Solid Edge part; units mm, degrees
sketch "Sketch1" plane through (0, 0, 0) normal (0, -1, 0) x (1, 0, 0)
  line L0 (0, 0) -> (115, 0)
  line L1 (115, 0) -> (115, 50)
  line L2 (115, 50) -> (0, 50)
  line L3 (0, 50) -> (0, 0)
  dimension "D1" = 115
extrude "Protrusion1" add sketch "Sketch1" against normal blind 50
fillet "Verrundung_2" radius 20 4 edges at (57.5, 50, 50) (57.5, 50, 0) (57.5, 0, 50) (57.5, 0, 0)
sketch "Sketch2" plane through (0, 25, 25) normal (-1, 0, 0) x (0, 0, -1)
  line L0 (-7.5, -7.5) -> (7.5, -7.5)
  line L1 (7.5, -7.5) -> (7.5, 7.5)
  line L2 (7.5, 7.5) -> (-7.5, 7.5)
  line L3 (-7.5, 7.5) -> (-7.5, -7.5)
  dimension "D1" = 7.5
extrude "Extrusionsausschnitt_5" cut sketch "Sketch2" against normal blind 15
chamfer "Fase_3" distance 2 angle 45 4 edges at (0, 25, 32.5) (0, 17.5, 25) (0, 25, 17.5) (0, 32.5, 25)
sketch "Sketch3" plane through (115, 25, 25) normal (1, 0, 0) x (0, 1, 0)
  line L0 (-7.5, -7.5) -> (7.5, -7.5)
  line L1 (7.5, -7.5) -> (7.5, 7.5)
  line L2 (7.5, 7.5) -> (-7.5, 7.5)
  line L3 (-7.5, 7.5) -> (-7.5, -7.5)
  dimension "D1" = 7.5
extrude "Extrusionsausprägung_2" add sketch "Sketch3" along normal blind 25
sketch "Sketch4" plane through (57.5, 25, 0) normal (0, 0, -1) x (-1, 0, 0)
  line L0 (-47.5, -17.5) -> (32.5, -17.5)
  line L1 (32.5, -17.5) -> (32.5, 17.5)
  line L2 (32.5, 17.5) -> (-47.5, 17.5)
  line L3 (-47.5, 17.5) -> (-47.5, -17.5)
  dimension "D1" = 32.5
  dimension "D2" = 32.5
extrude "Extrusionsausschnitt_6" cut sketch "Sketch4" against normal blind 20
sketch "Sketch5" plane through (65, 25, 20) normal (0, 0, -1) x (-1, 0, 0)
  line L0 (-40, 17.5) -> (40, 17.5)
  line L1 (40, 17.5) -> (40, -17.5)
  line L2 (40, -17.5) -> (-40, -17.5)
  line L3 (-40, -17.5) -> (-40, 17.5)
  line L4 (-34.5, 7) -> (-25.5, 7)
  line L5 (-25.5, 7) -> (-25.5, 16)
  line L6 (-25.5, 16) -> (-34.5, 16)
  line L7 (-34.5, 16) -> (-34.5, 7)
  line L8 (-34.5, -16) -> (-25.5, -16)
  line L9 (-25.5, -16) -> (-25.5, -7)
  line L10 (-25.5, -7) -> (-34.5, -7)
  line L11 (-34.5, -7) -> (-34.5, -16)
  line L12 (23.5, 7) -> (32.5, 7)
  line L13 (32.5, 7) -> (32.5, 16)
  line L14 (32.5, 16) -> (23.5, 16)
  line L15 (23.5, 16) -> (23.5, 7)
  line L16 (23.5, -16) -> (32.5, -16)
  line L17 (32.5, -16) -> (32.5, -7)
  line L18 (32.5, -7) -> (23.5, -7)
  line L19 (23.5, -7) -> (23.5, -16)
extrude "Extrusionsausschnitt_8" cut sketch "Sketch5" against normal blind 5
sketch "Sketch6" plane through (65, 42.5, 14.6938) normal (0, -1, 0) x (-1, 0, 0)
  line L0 (-40, -10.3062) -> (40, -10.3062)
  line L1 (40, -10.3062) -> (40, 10.3062)
  line L2 (40, 10.3062) -> (-40, 10.3062)
  line L3 (-40, 10.3062) -> (-40, -10.3062)
extrude "Extrusionsausschnitt_9" cut sketch "Sketch6" against normal blind 12
sketch "Sketch7" plane through (57.5, 50, 25) normal (0, 1, 0) x (-1, 0, 0)
  line L0 (32.5, 0) -> (45, -25)
  line L1 (45, -25) -> (32.5, -25)
  line L2 (32.5, -25) -> (32.5, 0)
extrude "Cutout1" cut sketch "Sketch7" against normal up to vertex (42.5 mm away)
fillet "Verrundung_3" radius 7.5 2 edges at (140, 25, 17.5) (140, 25, 32.5)
sketch "Sketch8" plane through (127.5, 32.5, 25) normal (0, 1, 0) x (-1, 0, 0)
  circle A0 centre (-5, 0) radius 2.05
extrude "Cutout2" cut sketch "Sketch8" against normal through all
chamfer "Fase_4" distance 1 angle 45 2 edges at (134.55, 32.5, 25) (132.5, 17.5, 22.95)
sketch "Sketch9" plane through (123.75, 25, 17.5) normal (0, 0, -1) x (-1, 0, 0)
  line L0 (8.75, -7.5) -> (8.75, 0)
  line L1 (8.75, 0) -> (-16.25, 0)
  line L2 (-16.25, 0) -> (-16.25, -7.5)
  line L3 (-16.25, -7.5) -> (8.75, -7.5)
extrude "Cutout3" cut sketch "Sketch9" against normal through all
sketch "Sketch10" plane through (95, 36.5, 20) normal (0, 0, -1) x (-1, 0, 0)
  line L0 (-4.5, 4.5) -> (62.5, 4.5)
  line L1 (62.5, 4.5) -> (62.5, -27.5)
  line L2 (62.5, -27.5) -> (-4.5, -27.5)
  line L3 (-4.5, -27.5) -> (-4.5, 4.5)
extrude "Cutout4" cut sketch "Sketch10" against normal up to vertex (5 mm away)
sketch "Sketch11" plane through (65, 28.75, 25) normal (0, 0, -1) x (-1, 0, 0)
  circle A0 centre (30, 13.25) radius 1.2
  circle A1 centre (-28, 13.25) radius 1.2
  circle A2 centre (-28, -9.75) radius 1.2
  circle A3 centre (30, -9.75) radius 1.2
  dimension "D1" = 30
extrude "Extrusionsausschnitt_14" cut sketch "Sketch11" against normal blind 10
sketch "Sketch12" plane through (65, 28.75, 25) normal (0, 0, -1) x (-1, 0, 0)
  line L0 (-31.5, 9.75) -> (-24.5, 9.75)
  line L1 (-24.5, 9.75) -> (-24.5, 16.75)
  line L2 (-24.5, 16.75) -> (-31.5, 16.75)
  line L3 (-31.5, 16.75) -> (-31.5, 9.75)
  line L4 (-31.5, -13.25) -> (-24.5, -13.25)
  line L5 (-24.5, -13.25) -> (-24.5, -6.25)
  line L6 (-24.5, -6.25) -> (-31.5, -6.25)
  line L7 (-31.5, -6.25) -> (-31.5, -13.25)
  line L8 (26.5, -13.25) -> (33.5, -13.25)
  line L9 (33.5, -13.25) -> (33.5, -6.25)
  line L10 (33.5, -6.25) -> (26.5, -6.25)
  line L11 (26.5, -6.25) -> (26.5, -13.25)
  line L12 (26.5, 9.75) -> (33.5, 9.75)
  line L13 (33.5, 9.75) -> (33.5, 16.75)
  line L14 (33.5, 16.75) -> (26.5, 16.75)
  line L15 (26.5, 16.75) -> (26.5, 9.75)
  circle A0 centre (-28, 13.25) radius 1.2
  circle A1 centre (-28, -9.75) radius 1.2
  circle A2 centre (30, -9.75) radius 1.2
  circle A3 centre (30, 13.25) radius 1.2
  dimension "D1" = 33.5
extrude "Extrusionsausprägung_3" add sketch "Sketch12" along normal blind 5
chamfer "Fase_5" distance 0.5 angle 45 4 edges at (94.2, 42, 20) (94.2, 19, 20) (36.2, 19, 20) (36.2, 42, 20)
properties part number "A6.A1.2" material "Nylon, allgemein"
Source: CAD feature listing. Evaluate the final solid. Frame: model axes, mm. A direction names the side the tool comes from. Give positions to 0.01 mm unless a question says otherwise; leave off trailing zeros. Loops run counter-clockwise (first coordinate to the right, second up) from the corner with the lowest first, then second, coordinate; pieces in that order, holes last. Notation, with made-up numbers: M 30,30 L 56,30 A15 cw 56,42 Z; hole C -32,44 d6. An arc over 180 degrees is marked long. Put each result on its own line as item: value.
Q1. Section A-A (x = 45). Return the cut outline in (y, z), and give its area (3 significant figures).
Response values:
outline: M 0,20 A20 ccw 7.5,4.39 L 7.5,25 L 50,25 L 50,30 A20 ccw 30,50 L 20,50 A20 ccw 0,30 Z
area: 1,200 mm²
Q2. Section B-B (y = 36). Return the cut outline in (x, z), and give its area (3 significant figures).
Response values:
outline: M 0,0.92 L 12.96,0.92 L 25,25 L 105,25 L 105,0.92 L 115,0.92 L 115,49.08 L 0,49.08 Z
area: 3,470 mm²
Q3. Line query: probe 1 along Y at (x, z) = (35, 31); probe 2 along X at (y, z) = (4, 28); probe 3 along X at (y, z) = (47.5, 21). Output: solid intervals per line, ascending. Write a range as [from, to].
Response values:
probe 1: y = [0.03, 17.8], [20.2, 40.8], [43.2, 49.97]
probe 2: x = [0, 115]
probe 3: x = [0, 23], [105, 115]
Q4. Reachability of faces 1 (the flat face through (58, 50, 26)), 2 (the flat face through (8, 25, 17.5)), 3 (the flat face through (38.5, 19, 23)), 4 (the flat face through (127, 32.5, 25)), 5 (the flat face through (93, 19, 35)) from +Z, -Z, +X, -X, +Y, -Y: full face, straight path, thin tool, end or side. Return the list, or none.
Response values:
face 1: +Z, -Z, +X, -X, +Y
face 2: -X
face 3: -Z, +Y
face 4: +Z, -Z, +X, +Y
face 5: -Z
Q5. Section C-C (z = 39.5). Return the cut outline in (x, y), and give its area (3 significant figures).
Response values:
outline: M 0,2.4 L 115,2.4 L 115,47.6 L 0,47.6 Z
area: 5,200 mm²
Q6. Mould query, pull axis X, two halves, no side actions, for faces 6 (the flat face through (105, 28, 12)), 7 (the flat face through (36, 44, 20)), 8 (the flat face through (6, 25, 0)), 9 (the cylindrical face through (137.862, 28.697, 30.245)). Classes: released by +X, released by -X, zero draft, split by the parting line, or undercut.
Response values:
face 6: undercut
face 7: undercut
face 8: zero draft
face 9: released by +X
Q7. Pin query (flat end, axial travel): P1, Ø1.9, axis at x = 35, y = 42, coming from the -Z side; P2, Ø10, axis at y = 9.5, z = 43, coming from the +X side; P3, Ø4, axis at x = 98.5, y = 33, coming from the -Z side; P4, Ø3, axis at x = 118, z = 39.5, coming from the +Y side. Return the tip coordinate at first contact, or that it passes through.
Response values:
P1: stops at z = 35
P2: stops at x = 115
P3: stops at z = 25
P4: passes through
